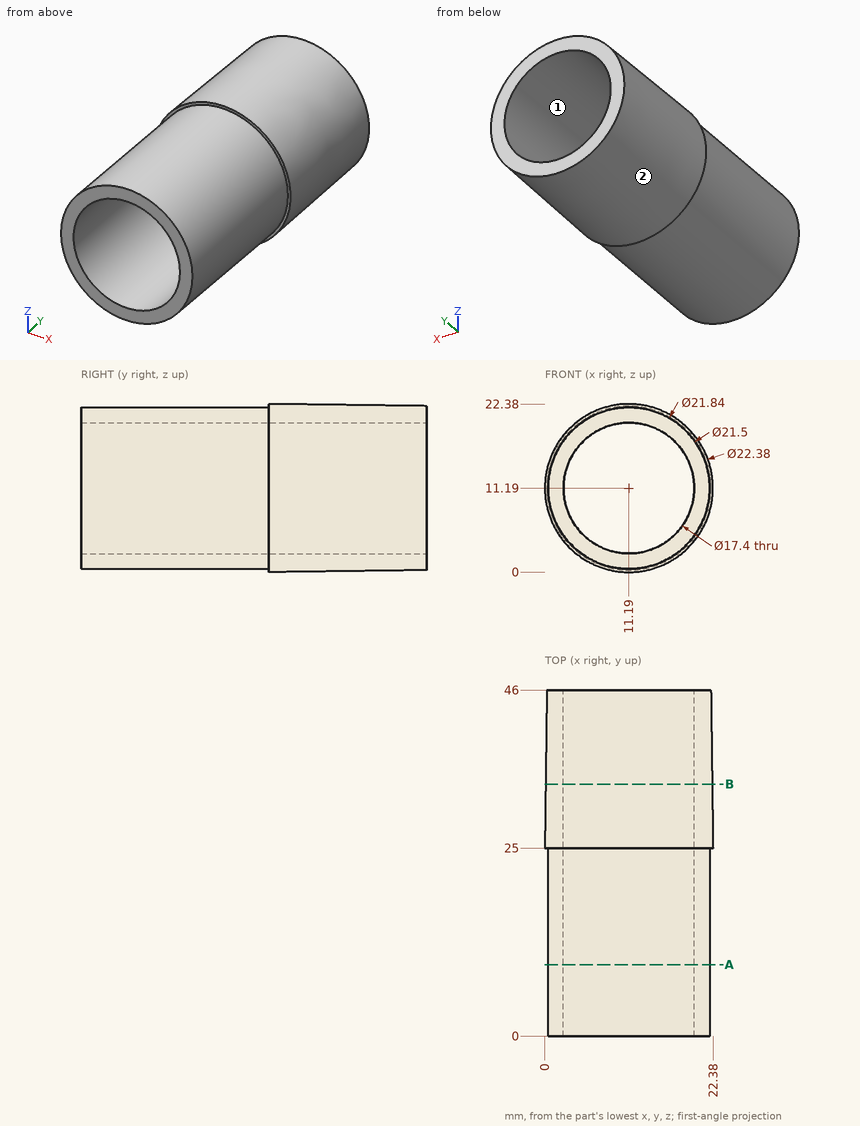
Job drawing, mm, ordinate dimensions from the low corner. One solid piece. Round coordinates to 2 decimals unless told otherwise and drop trailing zeros. Loops run counter-clockwise (first coordinate to the right, second up) from the corner with the lowest first, then second, coordinate; pieces in that order, holes last. Notation, with made-up numbers: M 51.25,6 L 76.25,6 A21 ccw 76.25,14 Z; hole C 52.5,79 d7. An arc over 180 degrees is marked long. One line per question, with ' | ' between items. Start each with the question number.
Item 1: Pin check, flat tips, straight feed: pin 1 Ø11 at (x, z) = (11, 12) entering from -Y; pin 2 Ø10 at (x, y) = (5.5, 35) entering from +Z; pin 3 Ø10 at (x, z) = (7.5, 5) entering from +Y; pin 4 Ø5 at (y, z) = (24, 6.5) entering from +X. Stop position of each tip, or through.
Item 2: Cut at A-A, the plane y = 9.5. Write the cut outline in (x, z).
Item 3: Cut at B-B, the plane y = 33.5. Write the cut outline in (x, z).
Item 4: Two-plate mould, pull along Z, no slides. Class the marked faces 1 and 2: pulls with the +Z half, pulls with the -Z half, needs draft (parallel to the pull), parting line crosses it, or undercut.
Item 5: Wall check: line 1 (Z direction, x = 11.19, y = 23); line 2 (X direction, y = 27, z = 14.75). Give the ranges that are in metal, low to high.
Responses:
1) pin 1: passes through | pin 2: stops at z = 22.24 | pin 3: stops at y = 46 | pin 4: stops at x = 22.12
2) outline: C 11.19,11.19 d21.5; hole C 11.19,11.19 d17.4
3) outline: C 11.19,11.19 d22.16; hole C 11.19,11.19 d17.4
4) face 1: undercut | face 2: parting line crosses it
5) line 1: z = 0.44 to 2.49, 19.89 to 21.94 | line 2: x = 0.61 to 3.25, 19.13 to 21.77
